Autodesk Inventor part; units mm, degrees
ref_plane "YZ Plane" through (0, 0, 0) normal (1, 0, 0) x (0, 1, 0)
ref_plane "XZ Plane" through (0, 0, 0) normal (0, 1, 0) x (-1, 0, 0)
ref_plane "XY Plane" through (0, 0, 0) normal (0, 0, 1) x (1, 0, 0)
sketch "Sketch_10" plane through (0, 0, 0) normal (0, 1, 0) x (-1, 0, 0)
  line L0 (21.2471, -13.0048) -> (21.2471, 13.0048)
  line L1 (21.2471, 13.0048) -> (3.0004, 13.0048)
  arc A0 (3.0004, 13.0048) -> (0, 10.0044) centre (3.0004, 10.0044) ccw
  line L2 (0, 10.0044) -> (0, -10.0044)
  arc A1 (0, -10.0044) -> (3.0004, -13.0048) centre (3.0004, -10.0044) ccw
  line L3 (3.0004, -13.0048) -> (21.2471, -13.0048)
extrude "Extrusion1" add sketch "Sketch_10" along normal blind 40.9956
sketch "Sketch_11" plane through (-21.2471, 0, 0) normal (1, 0, 0) x (0, 0, -1)
  arc A0 (-13.0048, 36.9951) -> (-10.0044, 33.9947) centre (-10.0044, 36.9951) ccw
  line L0 (-10.0044, 33.9947) -> (10.0044, 33.9947)
  arc A1 (10.0044, 33.9947) -> (13.0048, 36.9951) centre (10.0044, 36.9951) ccw
  line L1 (13.0048, 36.9951) -> (13.0048, 55.2418)
  line L2 (13.0048, 55.2418) -> (-13.0048, 55.2418)
  line L3 (-13.0048, 55.2418) -> (-13.0048, 36.9951)
extrude "Extrusion2" add sketch "Sketch_11" along normal blind 139.0142
sketch "Sketch_12" plane through (0, 0, 0) normal (0, 1, 0) x (-1, 0, 0)
  arc A0 (-96.52, 10.0044) -> (-99.5204, 13.0048) centre (-99.5204, 10.0044) ccw
  line L0 (-99.5204, 13.0048) -> (-117.7671, 13.0048)
  line L1 (-117.7671, 13.0048) -> (-117.7671, -13.0048)
  line L2 (-117.7671, -13.0048) -> (-99.5204, -13.0048)
  arc A1 (-99.5204, -13.0048) -> (-96.52, -10.0044) centre (-99.5204, -10.0044) ccw
  line L3 (-96.52, -10.0044) -> (-96.52, 10.0044)
extrude "Extrusion3" add sketch "Sketch_12" along normal blind 40.9956
sketch "Sketch_13" plane through (0, 23.0124, 0) normal (0, 1, 0) x (1, 0, 0)
  line L0 (12.1412, 10.0044) -> (12.1412, -10.0044)
  line L1 (-21.2471, 13.0048) -> (-21.2471, -13.0048)
  line L2 (-21.2471, -13.0048) -> (-3.0004, -13.0048)
  arc A0 (-3.0004, -13.0048) -> (0, -10.0044) centre (-3.0004, -10.0044) ccw
  line L3 (0, -10.0044) -> (0, 10.0044)
  arc A1 (0, 10.0044) -> (-3.0004, 13.0048) centre (-3.0004, 10.0044) ccw
  line L4 (-3.0004, 13.0048) -> (-21.2471, 13.0048)
revolve "Revolution1" add sketch "Sketch_13" angle 90 about axis through (12.1412, 23.0124, -10.0044) along (0, 0, -1)
sketch "Sketch_14" plane through (0, 23.0124, 0) normal (0, 1, 0) x (1, 0, 0)
  line L0 (84.3788, -10.0044) -> (84.3788, 10.0044)
  arc A0 (96.52, -10.0044) -> (99.5204, -13.0048) centre (99.5204, -10.0044) ccw
  line L1 (99.5204, -13.0048) -> (117.7671, -13.0048)
  line L2 (117.7671, -13.0048) -> (117.7671, 13.0048)
  line L3 (117.7671, 13.0048) -> (99.5204, 13.0048)
  arc A1 (99.5204, 13.0048) -> (96.52, 10.0044) centre (99.5204, 10.0044) ccw
  line L4 (96.52, 10.0044) -> (96.52, -10.0044)
revolve "Revolution2" add sketch "Sketch_14" angle 90 about axis through (84.3788, 23.0124, 10.0044) along (0, 0, 1)
sketch "Sketch_15" plane through (0, 0, 0) normal (0, 0, 1) x (1, 0, 0)
  line L0 (-33.9471, 81.9912) -> (-33.9471, 0)
  line L1 (-33.9471, 0) -> (-21.2471, 0)
  arc A0 (-19.4945, 15.0114) -> (-21.2471, 0) centre (51.2063, -0.851) ccw
  arc A1 (-9.9187, 34.0868) -> (-19.4945, 15.0114) centre (20.6584, 6.796) ccw
  arc A2 (3.0099, 40.9956) -> (-9.9187, 34.0868) centre (4.3058, 23.0194) ccw
  line L2 (3.0099, 40.9956) -> (93.5101, 40.9956)
  arc A3 (106.4387, 34.0868) -> (93.5101, 40.9956) centre (92.2142, 23.0194) ccw
  arc A4 (116.0145, 15.0114) -> (106.4387, 34.0868) centre (75.8616, 6.796) ccw
  arc A5 (117.7671, 0) -> (116.0145, 15.0114) centre (45.3137, -0.851) ccw
  line L3 (117.7671, 0) -> (130.4671, 0)
  line L4 (130.4671, 0) -> (130.4671, 81.9912)
  line L5 (130.4671, 81.9912) -> (-33.9471, 81.9912)
extrude "Extrusion4" cut sketch "Sketch_15" along normal mid plane 52.0192
sketch "Sketch_16" plane through (0, 0, 0) normal (0, 0, 1) x (1, 0, 0)
  line L0 (106.7689, 0) -> (106.7689, 40.9956)
  line L1 (106.7689, 40.9956) -> (113.2697, 40.9956)
  line L2 (113.2697, 40.9956) -> (113.2697, 6.0008)
  line L3 (113.2697, 6.0008) -> (111.0194, 6.0008)
  line L4 (111.0194, 6.0008) -> (111.0194, 0)
  line L5 (111.0194, 0) -> (106.7689, 0)
  line L6 (106.7689, 0) -> (106.7689, 40.9956)
revolve "Revolution3" cut sketch "Sketch_16" angle 360 about axis through (106.7689, 0, 0) along (0, -1, 0)
sketch "Sketch_17" plane through (0, 0, 0) normal (0, 0, 1) x (1, 0, 0)
  line L0 (-10.2489, 0) -> (-10.2489, 40.9956)
  line L1 (-10.2489, 40.9956) -> (-3.7481, 40.9956)
  line L2 (-3.7481, 40.9956) -> (-3.7481, 6.0008)
  line L3 (-3.7481, 6.0008) -> (-5.9984, 6.0008)
  line L4 (-5.9984, 6.0008) -> (-5.9984, 0)
  line L5 (-5.9984, 0) -> (-10.2489, 0)
  line L6 (-10.2489, 0) -> (-10.2489, 40.9956)
revolve "Revolution4" cut sketch "Sketch_17" angle 360 about axis through (-10.2489, 0, 0) along (0, -1, 0)
sketch "Sketch_18" plane through (0, 40.9956, 0) normal (0, 1, 0) x (1, 0, 0)
  line L0 (-33.9471, 25.7048) -> (-33.9471, -10.0013)
  line L1 (-33.9471, -10.0013) -> (-5.0206, -10.0013)
  arc A0 (-5.0206, -10.0013) -> (-3.0204, -8.001) centre (-5.0206, -8.001) ccw
  line L2 (-3.0204, -8.001) -> (-3.0204, 8.001)
  arc A1 (-3.0204, 8.001) -> (-5.0206, 10.0013) centre (-5.0206, 8.001) ccw
  line L3 (-5.0206, 10.0013) -> (-21.2471, 10.0013)
  line L4 (-21.2471, 10.0013) -> (-21.2471, 13.0048)
  line L5 (-21.2471, 13.0048) -> (117.7671, 13.0048)
  line L6 (117.7671, 13.0048) -> (117.7671, 10.0013)
  line L7 (117.7671, 10.0013) -> (101.5406, 10.0013)
  arc A2 (101.5406, 10.0013) -> (99.5404, 8.001) centre (101.5406, 8.001) ccw
  line L8 (99.5404, 8.001) -> (99.5404, -8.001)
  arc A3 (99.5404, -8.001) -> (101.5406, -10.0013) centre (101.5406, -8.001) ccw
  line L9 (101.5406, -10.0013) -> (130.4671, -10.0013)
  line L10 (130.4671, -10.0013) -> (130.4671, 25.7048)
  line L11 (130.4671, 25.7048) -> (-33.9471, 25.7048)
extrude "Extrusion5" cut sketch "Sketch_18" against normal blind 26.0032
properties part number "2061"
Geometry check sheet. Reference: the model listing, model coordinates, mm. A direction names the side the tool comes from. Round coordinates to 2 decimals unless told otherwise and drop trailing zeros. Write each loop counter-clockwise with the first axis right and the second up, starting at its lowest first coordinate (ties: lowest second). Pieces come first, ordered by that corner, then holes.
Item 1: Section check A-A (z = 0). Give the number of separate pieces and of enclosed holes in the cut face, plus the area to 3 significant figures.
Determined:
separate pieces: 3
enclosed holes: 0
area: 1,150 mm2
Item 2: Section check C-C (x = 108). Record the boundary of the cut face in (y, z).
Determined:
outline: (0, -13) - (32.23, -13) - (32.23, -10) - (14.99, -10) - (14.99, -6.38) - (6, -6.38) - (6, -4.07) - (0, -4.07) - close; (0, 4.07) - (6, 4.07) - (6, 6.38) - (14.99, 6.38) - (14.99, 10) - (32.23, 10) - (32.23, 13) - (0, 13) - close
Item 3: Access from +Z, -Z, +X, -X, +Y, -Y to the whole of each face (thin tool, end or side, straight path). Record for faces 1 (the face through (107, 24, 10.001)), 2 (the face through (96.52, 11, 0)), 3 (the face through (-17, 14.992, 0)), 4 (the face through (-0.856, 11.345, 12.103)), 5 (the face through (-4.048, 10.434, 1.953)).
Determined:
face 1: +X, +Y
face 2: +Z, -Z, -Y
face 3: -X, +Y
face 4: +Z, -Y
face 5: +Y
Item 4: Material ranges on line 1 along X through (y, z) = (12, 1); line 2 along Y through (x, z) = (61, 4.5); line 3 along Z through (x, y) = (109.5, 17), recorded low to high.
Determined:
line 1: x = -20.1 to -16.67, -3.83 to 0, 96.52 to 100.35, 113.19 to 116.62
line 2: y = 33.99 to 41
line 3: z = -13 to -10, 10 to 13
Item 5: Mould release check, pull along X, two halves, no side actions. Record for faces 6 (the face through (48, 40.996, 0)), 7 (the face through (-16.038, 25.048, 11.482)), 8 (the face through (97.422, 11.345, 12.149)): +X half, -X half, draft (parallel to the pull), parting line (faces both ways), or undercut.
Determined:
face 6: draft
face 7: -X half
face 8: undercut
Item 6: Go/stop test with flat-tipped pins: pin 1 Ø11.5 at (x, z) = (106.77, 0) entering from +Y; pin 2 Ø3 at (x, z) = (16, -8.5) entering from -Y; pin 3 Ø2 at (x, z) = (-1.5, -10) entering from -Y; pin 4 Ø5 at (y, z) = (29.5, -0.5) entering from -X. Record where each tip stops, or that it passes through.
Determined:
pin 1: stops at y = 6
pin 2: stops at y = 33.99
pin 3: stops at y = 0
pin 4: stops at x = -3.02
Item 7: Section check B-B (y = 21). Record the boundary of the cut face in (x, z).
Determined:
outline: (-17.79, -13) - (-3, -13) arc R3 ccw to (0, -10) - (0, 10) arc R3 ccw to (-3, 13) - (-17.79, 13) - (-17.79, 10) - (-5.02, 10) arc R2 cw to (-3.02, 8) - (-3.02, -8) arc R2 cw to (-5.02, -10) - (-17.79, -10) - close; (96.52, -10) arc R3 ccw to (99.52, -13) - (114.31, -13) - (114.31, -10) - (101.54, -10) arc R2 cw to (99.54, -8) - (99.54, 8) arc R2 cw to (101.54, 10) - (114.31, 10) - (114.31, 13) - (99.52, 13) arc R3 ccw to (96.52, 10) - close
Item 8: Section check D-D (x = 19). Record the boundary of the cut face in (y, z).
Determined:
outline: (33.99, -10) arc R3 ccw to (37, -13) - (41, -13) - (41, 13) - (37, 13) arc R3 ccw to (33.99, 10) - close
